```python
from build123d import *

# Parameters (mm, degrees)
F0_R     = 2.6
F0_R_2   = 10
F1_DEPTH = 5


with BuildPart() as f1:
    # F0 (on Top) → F1 (new body)
    with BuildSketch(Plane.XY):
        with BuildLine():
            Line((-33.964466, -47.5), (33.964466, -47.5))
            Line((33.964466, -47.5), (37.5, -43.964466))
            Line((37.5, -43.964466), (37.5, 42.5))
            ThreePointArc((37.5, 42.5), (36.035534, 46.035534), (32.5, 47.5))
            Line((32.5, 47.5), (-17.5, 47.5))
            ThreePointArc((-17.5, 47.5), (-21.035534, 46.035534), (-22.5, 42.5))
            Line((-22.5, 42.5), (-22.5, 32.5))
            ThreePointArc((-22.5, 32.5), (-23.964466, 28.964466), (-27.5, 27.5))
            Line((-27.5, 27.5), (-32.5, 27.5))
            ThreePointArc((-32.5, 27.5), (-36.035534, 26.035534), (-37.5, 22.5))
            Line((-37.5, 22.5), (-37.5, -43.964466))
            Line((-37.5, -43.964466), (-33.964466, -47.5))
        make_face()
        with Locations((-22.5, -37.5)):
            Circle(F0_R, mode=Mode.SUBTRACT)
        with Locations((22.5, -37.5)):
            Circle(F0_R, mode=Mode.SUBTRACT)
        with Locations((0, -9.5)):
            Circle(F0_R_2, mode=Mode.SUBTRACT)
    extrude(amount=F1_DEPTH)


solid = f1.part
```
Build history of the part. All positions in model axes, mm. A direction names the side the tool comes from. Give positions to 0.01 mm unless a question says otherwise; leave off trailing zeros. Loops run counter-clockwise (first coordinate to the right, second up) from the corner with the lowest first, then second, coordinate; pieces in that order, holes last.
Item 1: Slice it at C-C, the plane y = -37.5. List the corners of the cut face in (x, z), and give its area (3 significant figures).
Answers follow:
outline: (-37.5, 0) - (-25.1, 0) - (-25.1, 5) - (-37.5, 5) - close; (-19.9, 0) - (19.9, 0) - (19.9, 5) - (-19.9, 5) - close; (25.1, 0) - (37.5, 0) - (37.5, 5) - (25.1, 5) - close
area: 323 mm2
Item 2: Slice it at A-A, the plane y = -9.5. List the corners of the cut face in (x, z).
Answers follow:
outline: (-37.5, 0) - (-10, 0) - (-10, 5) - (-37.5, 5) - close; (10, 0) - (37.5, 0) - (37.5, 5) - (10, 5) - close
Item 3: Slice it at B-B, the plane x = 0. List the corners of the cut face in (y, z).
Answers follow:
outline: (-47.5, 0) - (-19.5, 0) - (-19.5, 5) - (-47.5, 5) - close; (0.5, 0) - (47.5, 0) - (47.5, 5) - (0.5, 5) - close
Item 4: Pull direction Y, two halves, no side cores. Call faces 1 (the face through (-37.5, -10, 2)), 2 (the face through (-21.3, -39.807, 2.465)), 3 (the face through (0, -47.5, 2)): released by +Y, released by -Y, zero draft, split by the parting line, or undercut.
Answers follow:
face 1: zero draft
face 2: undercut
face 3: released by -Y
Item 5: Which spindle directions (+Z, -Z, +X, -X, +Y, -Y) get a long thin tool onto all of the face, cutting with end or side? Do faces 4 (the face through (-30, 27.5, 2)), 5 (the face through (36.07, 46, 2.46)). Say none if no direction does.
Answers follow:
face 4: +Z, -Z, -X, +Y
face 5: +Z, -Z, +X, +Y
Item 6: Drill centre lines: line 1 (Y direction, x = 22.5, z = 1.15); line 2 (X direction, y = -10, z = 4.45); line 3 (Y direction, x = 7.5, z = 0.5). Where is each one in solid material? Low to high.
Answers follow:
line 1: y = -47.5 to -40.1, -34.9 to 47.5
line 2: x = -37.5 to -9.99, 9.99 to 37.5
line 3: y = -47.5 to -16.11, -2.89 to 47.5
Item 7: Flat gauge pins, fed straight in: pin 1 (4 mm diameter, centred on x = 22.5, y = -37.5, fed in from -Z); pin 2 (1.5 mm diameter, centred on y = 36, z = 3, fed in from -X). Where does each tip first touch, or does it go through?
Answers follow:
pin 1: passes through
pin 2: stops at x = -22.5
Item 8: Slice it at D-D, the plane z = 2.6. List the corners of the cut face in (x, y).
Answers follow:
outline: (-37.5, -43.96) - (-33.96, -47.5) - (33.96, -47.5) - (37.5, -43.96) - (37.5, 42.5) arc R5 ccw to (32.5, 47.5) - (-17.5, 47.5) arc R5 ccw to (-22.5, 42.5) - (-22.5, 32.5) arc R5 cw to (-27.5, 27.5) - (-32.5, 27.5) arc R5 ccw to (-37.5, 22.5) - close; hole circle Ø5.2 at (-22.5, -37.5); hole circle Ø20 at (0, -9.5); hole circle Ø5.2 at (22.5, -37.5)
